Autodesk Inventor part; units mm, degrees
ref_plane "YZ Plane" through (0, 0, 0) normal (1, 0, 0) x (0, 1, 0)
ref_plane "XZ Plane" through (0, 0, 0) normal (0, 1, 0) x (-1, 0, 0)
ref_plane "XY Plane" through (0, 0, 0) normal (0, 0, 1) x (1, 0, 0)
sketch "Sketch1" plane through (0, 0, 0) normal (0, 0, 1) x (1, 0, 0)
  line L0 (-11, -17.5) -> (11, -17.5)
  line L1 (11, -17.5) -> (11, 17.5)
  line L2 (11, 17.5) -> (-11, 17.5)
  line L3 (-11, 17.5) -> (-11, -17.5)
  line L4 (-11, -17.5) -> (11, 17.5) construction
  line L5 (11, -17.5) -> (-11, 17.5) construction
  point P0 (0, 0)
  dimension "d0" = 22
  dimension "d1" = 35
extrude "Extrusion1" add sketch "Sketch1" along normal blind 10
sketch "Sketch2" plane through (0, 0, 10) normal (0, 0, 1) x (1, 0, 0)
  line L0 (-11, -17.5) -> (19, -17.5)
  line L1 (19, -17.5) -> (19, -2.5)
  line L2 (19, -2.5) -> (-11, -2.5)
  line L3 (-11, -2.5) -> (-11, -17.5)
  point P0 (0, 0)
  dimension "d4" = 30
  dimension "d5" = 15
extrude "Extrusion2" cut sketch "Sketch2" against normal blind 8
sketch "Sketch4" plane through (0, 0, 2) normal (0, 0, 1) x (1, 0, 0)
  circle A0 centre (-7.5, -12.5) radius 2.45
  circle A1 centre (7.5, -12.5) radius 2.45
  line L0 (11, -17.5) -> (-11, -17.5)
  point P0 (0, 0)
  dimension "d12" = 4.9
  dimension "d13" = 4.9
  dimension "d14" = 15
  dimension "d15" = 7.5
  dimension "d16" = 5
  dimension "d17" = 5
hole "Hole1" at (-7.5, -12.5, 2) at (7.5, -12.5, 2) direction (0, 0, -1) diameter 4.6 end through all
sketch "Sketch5" plane through (-11, 17.5, 0) normal (0, 1, 0) x (1, 0, 0)
  circle A0 centre (7.75, -5.5) radius 2.95
  circle A1 centre (14.25, -5.5) radius 2.95
  line L0 (22, -10) -> (0, -10)
  point P0 (11, 0)
  dimension "d25" = 5.9
  dimension "d26" = 5.9
  dimension "d27" = 6.5
  dimension "d28" = 3.25
  dimension "d29" = 4.5
  dimension "d30" = 4.5
extrude "Extrusion8" cut sketch "Sketch5" against normal blind 8
sketch "Sketch9" plane through (-11, -2.5, 2) normal (0, -1, 0) x (1, 0, 0)
  circle A0 centre (7.75, 3.5) radius 2.95
  circle A1 centre (7.75, 3.5) radius 1.25
  point P0 (11, -2)
  dimension "d45" = 2.5
extrude "Extrusion9" cut sketch "Sketch9" against normal up to next contours A1
sketch "Sketch13" plane through (-11, -2.5, 10) normal (0, -1, 0) x (1, 0, 0)
  circle A0 centre (14.25, -4.5) radius 2.95
  circle A1 centre (14.25, -4.5) radius 1.25
  point P0 (11, -10)
  dimension "d58" = 2.5
extrude "Extrusion13" cut sketch "Sketch13" against normal up to next contours A1
sketch "Sketch14" plane through (0, 0, 2) normal (0, 0, 1) x (1, 0, 0)
  line L0 (-11, -2.5) -> (11, -2.5)
  line L1 (-1, -2.5) -> (1, -2.5)
  line L2 (1, -2.5) -> (1, -17.5)
  line L3 (1, -17.5) -> (-1, -17.5)
  line L4 (-1, -17.5) -> (-1, -2.5)
  point P0 (0, 0)
  dimension "d61" = 2
  dimension "d62" = 15
  dimension "d63" = 1
extrude "Extrusion14" add sketch "Sketch14" along normal blind 8
equation "\"d30\" = d29"
properties part number "HVcup"
The model under review builds one solid part; all positions refer to its coordinate system, in mm. A direction names the side the tool comes from. Give positions to 0.01 mm unless a question says otherwise; leave off trailing zeros. Order: outer loops, then holes, each group sorted by start corner. A loop starts at its lowest first (then second) coordinate and runs counter-clockwise, first axis right, second up. Notation, with made-up numbers: M 88.5,-13.5 L 120.5,-13.5 A10 ccw 120.5,-3.5 Z; hole C -22.5,23 d11. An arc over 180 degrees is marked long. Use one line per item in the form item = value. Start each with the question number.
Item 1: Insertion check: pin 1 Ø3 at (x, z) = (-3.25, 5.5) entering from -Y; pin 2 Ø6 at (x, y) = (7.5, -12.5) entering from +Z; pin 3 Ø4 at (y, z) = (-13.5, 7) entering from -X. Each pin has a flat end and moves straight along its axis. Give the tip position at first contact, or say it passes through.
Item 2: We need section C-C on y = 6. Give the boundary of the cut face in (x, z), plus the area to 3 significant figures.
Item 3: We need section B-B on y = -12.5. Give the boundary of the cut face in (x, z), plus the area to 3 significant figures.
Item 4: To check wall thickness, follow line 1 along X through (y, z) = (15, 5.5); line 2 along X through (y, z) = (-12.5, 1.55); line 3 along Z through (x, y) = (3.25, 3.25). State the ranges of each line that lie inside material, in increasing order. Write a range as from..to.
Item 5: We need section D-D on x = -3.25. Give the boundary of the cut face in (y, z), plus the area to 3 significant figures.
Item 6: For faces 4 (the flat face through (6, -2.5, 6)), 5 (the cylindrical face through (-2.673, 3.416, 4.391)), 6 (the flat face through (-3, 9.5, 7)), 7 (the flat face through (-11, 4, 4)), 8 (the flat face through (-1, -10, 6)), list the 3-axis set-ups (+Z, -Z, +X, -X, +Y, -Y) from which the entire face can be reached by the end or side of a thin tool; tool diameter is ignored.
Item 7: We need section A-A on x = 7.5. Give the boundary of the cut face in (y, z), plus the area to 3 significant figures.
Item 8: The part is to be moulded in two halves that separate along X. For faces 1 (the flat face through (0, 8, 10)), 2 (the flat face through (5, 9.5, 5)), 3 (the flat face through (1, -10, 6)), say which applies: pulls with the +X half, pulls with the -X half, needs draft (parallel to the pull), parting line crosses it, or undercut.
Completed:
q1.pin_1 = -2.5
q1.pin_2 = 2
q1.pin_3 = -1
q2.outline = M -11,0 L 11,0 L 11,10 L -11,10 Z; hole C -3.25,5.5 d2.5; hole C 3.25,5.5 d2.5
q2.area = 210 mm²
q3.outline = M -11,0 L -9.8,0 L -9.8,2 L -11,2 Z; M -5.2,0 L 5.2,0 L 5.2,2 L 1,2 L 1,10 L -1,10 L -1,2 L -5.2,2 Z; M 9.8,0 L 11,0 L 11,2 L 9.8,2 Z
q3.area = 41.6 mm²
q4.line_1 = -11..-6.2, -0.3..0.3, 6.2..11
q4.line_2 = -11..-9.8, -5.2..5.2, 9.8..11
q4.line_3 = 0..4.25, 6.75..10
q5.outline = M -17.5,0 L 17.5,0 L 17.5,2.55 L 9.5,2.55 L 9.5,4.25 L -2.5,4.25 L -2.5,2 L -17.5,2 Z; M -2.5,6.75 L 9.5,6.75 L 9.5,8.45 L 17.5,8.45 L 17.5,10 L -2.5,10 Z
q5.area = 153 mm²
q6.face_4 = +Z, +X, -Y
q6.face_5 = +Y, -Y
q6.face_6 = +Y
q6.face_7 = +Z, -Z, -X, +Y, -Y
q6.face_8 = +Z, -X, -Y
q7.outline = M -17.5,0 L -14.8,0 L -14.8,2 L -17.5,2 Z; M -10.2,0 L 17.5,0 L 17.5,10 L -2.5,10 L -2.5,2 L -10.2,2 Z
q7.area = 221 mm²
q8.face_1 = needs draft
q8.face_2 = undercut
q8.face_3 = pulls with the +X half
